Here's how the part is built. I have some questions about the finished solid (model axes, mm). Coordinates: 2 decimals unless noted, no trailing zeros. Loops run counter-clockwise (first coordinate to the right, second up) from the corner with the lowest first, then second, coordinate; pieces in that order, holes last.
from build123d import *

# Parameters (mm, degrees)
BOSS_EXTRUDE1_DEPTH = 34.1
CUT_EXTRUDE1_DEPTH  = 7


with BuildPart() as part:
    # Sketch1 → Boss-Extrude1 (new body, symmetric)
    with BuildSketch(Plane.XY):
        with BuildLine():
            Line((0, 0), (-60.568627866, 0))
            ThreePointArc((-60.568627866, 0), (-61.957942591, 0.561318453), (-62.567409324, 1.930195406))
            Line((-62.567409324, 1.930195406), (-63.623195406, 32.161524241))
            ThreePointArc((-63.623195406, 32.161524241), (-63.087125173, 33.595321457), (-61.694218542, 34.230110294))
            Line((-61.694218542, 34.230110294), (-59.693, 34.3))
            Line((-59.693, 34.3), (-59.658097703, 33.300609271))
            Line((-59.658097703, 33.300609271), (-61.659316244, 33.230719565))
            ThreePointArc((-61.659316244, 33.230719565), (-62.35576956, 32.913325146), (-62.623804676, 32.196426538))
            Line((-62.623804676, 32.196426538), (-61.568018595, 1.965097703))
            ThreePointArc((-61.568018595, 1.965097703), (-61.263285228, 1.280659226), (-60.568627866, 1))
            Line((-60.568627866, 1), (0, 1))
            Line((0, 1), (60.568627866, 1))
            ThreePointArc((60.568627866, 1), (61.263285228, 1.280659226), (61.568018595, 1.965097703))
            Line((61.568018595, 1.965097703), (62.623804676, 32.196426538))
            ThreePointArc((62.623804676, 32.196426538), (62.35576956, 32.913325146), (61.659316244, 33.230719565))
            Line((61.659316244, 33.230719565), (59.658097703, 33.300609271))
            Line((59.658097703, 33.300609271), (59.693, 34.3))
            Line((59.693, 34.3), (61.694218542, 34.230110294))
            ThreePointArc((61.694218542, 34.230110294), (63.087125173, 33.595321457), (63.623195406, 32.161524241))
            Line((63.623195406, 32.161524241), (62.567409324, 1.930195406))
            ThreePointArc((62.567409324, 1.930195406), (61.957942591, 0.561318453), (60.568627866, 0))
            Line((60.568627866, 0), (0, 0))
        make_face()
    extrude(amount=BOSS_EXTRUDE1_DEPTH, both=True)

    # Sketch2 → Cut-Extrude1 (cut)
    with BuildSketch(Plane(origin=(62.423864353, -2.180064512, 0), x_dir=(0, 0, -1), z_dir=(0.999390729, -0.034902297, 0))):
        Polygon((-34.1, 36.362524836), (-29.1, 36.362524836), (-34.1, 30.162524836), align=None)
    cut_extrude1 = extrude(amount=-CUT_EXTRUDE1_DEPTH, mode=Mode.SUBTRACT)

    # Mirror1: Cut-Extrude1 across plane
    add(cut_extrude1.mirror(Plane(origin=(0, 0, 0), x_dir=(0, 0, 1), z_dir=(1, 0, 0))), mode=Mode.SUBTRACT)


solid = part.part
Q1. Suppose I cut it at B-B on y = 15. Write out the boundary of the cut face in (x, z).
Q2. Suppose I cut it at A-A on z = 8.5. Write out the boundary of the cut face in (x, y), and give its area (3 significant figures).
Q3. Please list where these lines run through material, in increasing order: probe 1 along X at (y, z) = (2, -15); probe 2 along X at (y, z) = (31.5, -10.5); probe 3 along Y at (x, z) = (-16, -23).
Q4. Suppose I cut it at C-C on x = 36. Write out the boundary of the cut face in (y, z).
Q5. Will this pin go through, and if not, where does the flat tip stop? P1, Ø6, axis at x = 29, z = -15.5, coming from the +Y side.
Check values:
1. outline: (-63.02, -34.1) - (-62.02, -34.1) - (-62.02, 34.1) - (-63.02, 34.1) - close; (62.02, -34.1) - (63.02, -34.1) - (63.02, 34.1) - (62.02, 34.1) - close
2. outline: (-63.62, 32.16) - (-62.57, 1.93) arc R2 ccw to (-60.57, 0) - (60.57, 0) arc R2 ccw to (62.57, 1.93) - (63.62, 32.16) arc R2 ccw to (61.69, 34.23) - (59.69, 34.3) - (59.66, 33.3) - (61.66, 33.23) arc R1 cw to (62.62, 32.2) - (61.57, 1.97) arc R1 cw to (60.57, 1) - (-60.57, 1) arc R1 cw to (-61.57, 1.97) - (-62.62, 32.2) arc R1 cw to (-61.66, 33.23) - (-59.66, 33.3) - (-59.69, 34.3) - (-61.69, 34.23) arc R2 ccw to start
2. area: 195 mm2
3. probe 1: x = -62.57 to -61.57, 61.57 to 62.57
3. probe 2: x = -63.6 to -62.6, 62.6 to 63.6
3. probe 3: y = 0 to 1
4. outline: (0, -34.1) - (1, -34.1) - (1, 34.1) - (0, 34.1) - close
5. P1: stops at y = 1
